For this review, take the finished solid that the model builds, in its own axes (mm). Face numbers are marked on the shaded views. A direction names the side the tool comes from. Give positions to 0.01 mm unless a question says otherwise; leave off trailing zeros. Write each loop counter-clockwise with the first axis right and the second up, starting at its lowest first coordinate (ties: lowest second). Pieces come first, ordered by that corner, then holes. Notation, with made-up numbers: M 40,29.5 L 50,29.5 A14 cw 50,47.5 Z; hole C 21.5,31.5 d7. An arc over 180 degrees is marked long. Answer as a JSON object with one key per item and string values. Group by question number.
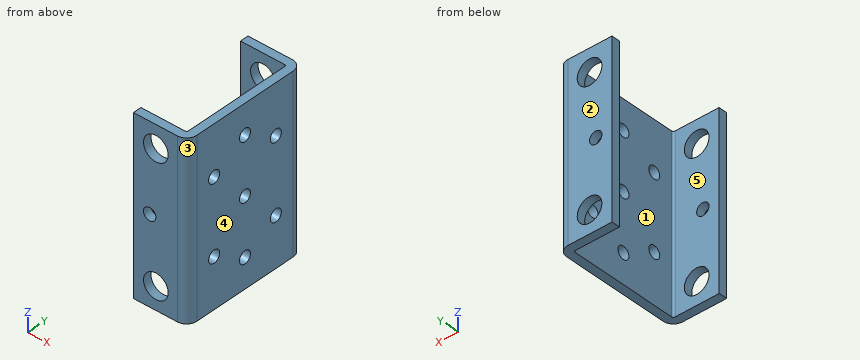
```python
from build123d import *

# Parameters (mm, degrees)
SKETCH11_W                     = 3.4
SKETCH11_H                     = 52
BASE_FLANGE3_DEPTH             = 70
EDGE_FLANGE1_STRIP_W           = 15.1
EDGE_FLANGE1_STRIP_H           = 3.4
EDGE_FLANGE1_STRIP_CUT_DEPTH   = 70
EDGE_FLANGE1_STRIP_2_W         = 15.1
EDGE_FLANGE1_STRIP_2_H         = 3.4
EDGE_FLANGE1_STRIP_CUT_2_DEPTH = 70
EDGE_FLANGE1_DEPTH             = 70
EDGE_FLANGE1_BEND_DEPTH        = 70
CUT_EXTRUDE1_DEPTH             = 89.011135659
CUT_EXTRUDE1_DEPTH_BACK        = 89.011135659
SKETCH25_R                     = 2.5
SKETCH25_R_2                   = 5
SKETCH23_R                     = 2.5
CUT_EXTRUDE2_DEPTH             = 77.954272136


# Sheet-metal steps are written as plain solids
with BuildPart() as part:
    # Sketch11 → Base-Flange3 (new body)
    with BuildSketch(Plane.XY):
        with Locations((-1.7, 0)):
            Rectangle(SKETCH11_W, SKETCH11_H)
    extrude(amount=BASE_FLANGE3_DEPTH)

    # Edge-Flange1 strip (across the edge) → Edge-Flange1 strip cut (cut)
    with BuildSketch(Plane(origin=(-3.4, 26, 70), x_dir=(0, -1, 0), z_dir=(0, 0, -1))):
        with Locations((-3.4, -1.7)):
            Rectangle(EDGE_FLANGE1_STRIP_W, EDGE_FLANGE1_STRIP_H)
    extrude(amount=EDGE_FLANGE1_STRIP_CUT_DEPTH, mode=Mode.SUBTRACT)

    # Edge-Flange1 strip 2 (across the edge) → Edge-Flange1 strip cut 2 (cut)
    with BuildSketch(Plane(origin=(-3.4, -26, 0), x_dir=(0, 1, 0), z_dir=(0, 0, 1))):
        with Locations((-3.4, -1.7)):
            Rectangle(EDGE_FLANGE1_STRIP_2_W, EDGE_FLANGE1_STRIP_2_H)
    extrude(amount=EDGE_FLANGE1_STRIP_CUT_2_DEPTH, mode=Mode.SUBTRACT)

    # Edge-Flange1 section (across the edge) → Edge-Flange1 (add)
    with BuildSketch(Plane(origin=(-3.4, 26, 70), x_dir=(0, -1, 0), z_dir=(0, 0, -1))):
        with BuildLine():
            Line((0, 0.75), (0, 18.6))
            Line((0, 18.6), (3.4, 18.6))
            Line((3.4, 18.6), (3.4, 0.75))
            ThreePointArc((3.4, 0.75), (3.619669914, 0.219669914), (4.15, 0))
            Line((4.15, 0), (4.15, -3.4))
            ThreePointArc((4.15, -3.4), (1.215506858, -2.184493142), (0, 0.75))
        make_face()
    extrude(amount=EDGE_FLANGE1_DEPTH)

    # Edge-Flange1 section 2 (across the edge) → Edge-Flange1 bend (add)
    with BuildSketch(Plane(origin=(-3.4, -26, 0), x_dir=(0, 1, 0), z_dir=(0, 0, 1))):
        with BuildLine():
            Line((0, 0.75), (0, 18.6))
            Line((0, 18.6), (3.4, 18.6))
            Line((3.4, 18.6), (3.4, 0.75))
            ThreePointArc((3.4, 0.75), (3.619669914, 0.219669914), (4.15, 0))
            Line((4.15, 0), (4.15, -3.4))
            ThreePointArc((4.15, -3.4), (1.215506858, -2.184493142), (0, 0.75))
        make_face()
    extrude(amount=EDGE_FLANGE1_BEND_DEPTH)

    # Sketch25 → Cut-Extrude1 (cut, two sides: drawn at the far end of the back side and taken through both)
    with BuildSketch(Plane.XZ.offset(-22.6).offset(-CUT_EXTRUDE1_DEPTH_BACK)):
        with Locations((-15.4, 35)):
            Circle(SKETCH25_R)
        with Locations((-12.9, 9.1)):
            Circle(SKETCH25_R_2)
        with Locations(Location((-12.9, 60.9, 0), (0, 0, 180))):
            Circle(SKETCH25_R_2)
    extrude(amount=CUT_EXTRUDE1_DEPTH + CUT_EXTRUDE1_DEPTH_BACK, mode=Mode.SUBTRACT)

    # Sketch23 → Cut-Extrude2 (cut, through all)
    with BuildSketch(Plane.ZY.offset(3.4)):
        with Locations(Location((20, -14, 0), (0, 0, 270))):
            Circle(SKETCH23_R)
        with Locations(Location((50, -14, 0), (0, 0, 270))):
            Circle(SKETCH23_R)
        with Locations(Location((20, 14, 0), (0, 0, 90))):
            Circle(SKETCH23_R)
        with Locations(Location((50, 14, 0), (0, 0, 270))):
            Circle(SKETCH23_R)
        with Locations(Location((35, 0, 0), (0, 0, 270))):
            Circle(SKETCH23_R)
        with Locations(Location((58, 0, 0), (0, 0, 270))):
            Circle(SKETCH23_R)
        with Locations(Location((12, 0, 0), (0, 0, 90))):
            Circle(SKETCH23_R)
    extrude(amount=-CUT_EXTRUDE2_DEPTH, mode=Mode.SUBTRACT)


solid = part.part
```
Item 1: Draft analysis for pull direction Y (two halves, no side actions). For the marked faces 3, 4 and 5, state which applies: released by +Y, released by -Y, zero draft, split by the parting line, or undercut.
Item 2: Insertion check: P1, Ø6.5, axis at y = 0, z = 35, coming from the -X side; P2, Ø12, axis at x = -13.5, y = -6.5, coming from the -Z side. Each pin has a flat end and moves straight along its axis. Give the tip position at first contact, or say it passes through.
Item 3: Consider section B-B (x = -5.75). Give the boundary of the cut face in (y, z).
Item 4: Consider section D-D (y = 14). Give the boundary of the cut face in (x, z), plus the area to 3 significant figures.
Item 5: Consider section A-A (z = 50). Give the boundary of the cut face in (x, y), plus the area to 3 significant figures.
Item 6: To check wall thickness, follow probe 1 along Z at (x, y) = (-2.4, -14); probe 2 along Y at (x, z) = (-9.25, 19.5); probe 3 along X at (y, z) = (-23.65, 9.1). State the ranges of each line that lie inside material, in increasing order.
Item 7: Machinability: for the marked faces 1 and 2, which of the approach directions +Z, -Z, +X, -X, +Y, -Y give a long, thin tool a straight path to every point of the face, cutting with its end or side? Answer none if there is none.
Item 8: Consider section C-C (y = -0.5). Give the boundary of the cut face in (x, z), plus the area to 3 significant figures.
Result set:
{
 "1": {"face 3": "released by -Y", "face 4": "zero draft", "face 5": "undercut"},
 "2": {"P1": "stops at x = -3.4", "P2": "passes through"},
 "3": {"outline": "M -26,0 L -22.6,0 L -22.6,70 L -26,70 Z; M 22.6,0 L 26,0 L 26,70 L 22.6,70 Z"},
 "4": {"outline": "M -3.4,0 L 0,0 L 0,17.5 L -3.4,17.5 Z; M -3.4,22.5 L 0,22.5 L 0,47.5 L -3.4,47.5 Z; M -3.4,52.5 L 0,52.5 L 0,70 L -3.4,70 Z", "area": "204 mm^2"},
 "5": {"outline": "M -22,-26 L -4.15,-26 A4.15 ccw 0,-21.85 L 0,-16.5 L -3.4,-16.5 L -3.4,-21.85 A0.75 cw -4.15,-22.6 L -22,-22.6 Z; M -22,22.6 L -4.15,22.6 A0.75 cw -3.4,21.85 L -3.4,16.5 L 0,16.5 L 0,21.85 A4.15 ccw -4.15,26 L -22,26 Z; M -3.4,-11.5 L 0,-11.5 L 0,11.5 L -3.4,11.5 Z", "area": "262 mm^2"},
 "6": {"probe 1": "z = 0 to 17.5, 22.5 to 47.5, 52.5 to 70", "probe 2": "y = -26 to -22.6, 22.6 to 26", "probe 3": "x = -22 to -17.9, -7.9 to -0.41"},
 "7": {"face 1": "+Z, -Z, -X", "face 2": "+Z, -Z, +X, -X, +Y"},
 "8": {"outline": "M -3.4,0 L 0,0 L 0,9.55 L -3.4,9.55 Z; M -3.4,14.45 L 0,14.45 L 0,32.55 L -3.4,32.55 Z; M -3.4,37.45 L 0,37.45 L 0,55.55 L -3.4,55.55 Z; M -3.4,60.45 L 0,60.45 L 0,70 L -3.4,70 Z", "area": "188 mm^2"}
}
